from build123d import *

# Parameters (mm, degrees)
SKETCH1_W           = 110
SKETCH1_H           = 160
BOSS_EXTRUDE1_DEPTH = 3
SKETCH2_W           = 3
SKETCH2_H           = 15
BOSS_EXTRUDE2_DEPTH = 20
FILLET1_R           = 5
SKETCH3_R           = 3
CUT_EXTRUDE1_DEPTH  = 120
CUT_EXTRUDE2_DEPTH  = 10


with BuildPart() as part:
    # Sketch1 → Boss-Extrude1 (new body)
    with BuildSketch(Plane.XY):
        with Locations((55, 80)):
            Rectangle(SKETCH1_W, SKETCH1_H)
    extrude(amount=BOSS_EXTRUDE1_DEPTH)

    # Sketch2 → Boss-Extrude2 (add)
    with BuildSketch(Plane(origin=(0, 0, 0), x_dir=(-1, 0, 0), z_dir=(0, 0, -1))):
        with Locations((-4.5, 122.5)):
            Rectangle(SKETCH2_W, SKETCH2_H)
        with Locations((-4.5, 37.5)):
            Rectangle(SKETCH2_W, SKETCH2_H)
        with Locations((-105.5, 37.5)):
            Rectangle(SKETCH2_W, SKETCH2_H)
        with Locations((-105.5, 122.5)):
            Rectangle(SKETCH2_W, SKETCH2_H)
    extrude(amount=BOSS_EXTRUDE2_DEPTH)

    # Fillet1
    fillet1_edges = [part.edges().sort_by_distance(p)[0] for p in [
        (6, 122.5, 0),
        (6, 37.5, 0),
        (104, 37.5, 0),
        (104, 122.5, 0),
    ]]
    fillet(fillet1_edges, radius=FILLET1_R)

    # Sketch3 → Cut-Extrude1 (cut)
    with BuildSketch(Plane(origin=(107, 0, 0), x_dir=(0, 0, -1), z_dir=(1, 0, 0))):
        with Locations((10, 122.5)):
            Circle(SKETCH3_R)
        with Locations((10, 37.5)):
            Circle(SKETCH3_R)
    extrude(amount=-CUT_EXTRUDE1_DEPTH, mode=Mode.SUBTRACT)

    # Sketch4 → Cut-Extrude2 (cut)
    with BuildSketch(Plane(origin=(0, 0, 0), x_dir=(-1, 0, 0), z_dir=(0, 0, -1))):
        Polygon((-97.404603448, 115.083332467), (-71.456820791, 149.11710788), (-97.404603448, 149.11710788), align=None)
        Polygon((-39.377270954, 115.240473699), (-75.208928564, 132.650284128), (-97.404603448, 103.53786924), (-97.404603448, 79.025613644), align=None)
        Polygon((-12.834970583, 149.11710788), (-62.654412981, 149.11710788), (-70.879295193, 138.329141999), (-12.834970583, 110.126687653), align=None)
        Polygon((-12.834970583, 56.494500283), (-12.834970583, 102.344156626), (-31.943432736, 111.628536023), (-63.844562164, 91.719040132), align=None)
        Polygon((-70.31535921, 87.68061549), (-97.404603448, 70.774217299), (-97.404603448, 39.706571637), (-44.85383039, 70.098223458), align=None)
        Polygon((-78.83079022, 42.362019492), (-97.404603448, 31.620239081), (-97.404603448, 10.88289212), (-40.243023437, 10.88289212), align=None)
        Polygon((-12.834970583, 10.88289212), (-12.834970583, 47.98768369), (-38.481002615, 65.697483931), (-72.350817961, 46.109577315), (-29.169217126, 10.88289212), align=None)
    extrude(amount=-CUT_EXTRUDE2_DEPTH, mode=Mode.SUBTRACT)


solid = part.part
Work out the finished part from the listing and answer in its coordinate system (mm). A direction names the side the tool comes from. Give positions to 0.01 mm unless a question says otherwise; leave off trailing zeros. Write each loop counter-clockwise with the first axis right and the second up, starting at its lowest first coordinate (ties: lowest second). Pieces come first, ordered by that corner, then holes.
Q1. For a pull along X with two mould halves and no side action, classify faces 1 (the face through (102, 123, -1)), 2 (the face through (37, 149.117, 1)), 3 (the face through (4.521, 40.474, -9.609)), 4 (the face through (3, 34, -10)) as released by +X, released by -X, zero draft, split by the parting line, or undercut.
Answer:
face 1: undercut
face 2: undercut
face 3: zero draft
face 4: released by -X
Q2. The part is cut by section D-D on y = 141. Give the vertices of the cut face in (x, z).
Answer:
outline: (0, 0) - (12.83, 0) - (12.83, 3) - (0, 3) - close; (68.84, 0) - (77.65, 0) - (77.65, 3) - (68.84, 3) - close; (97.4, 0) - (110, 0) - (110, 3) - (97.4, 3) - close
Q3. The part is cut by section B-B on x = 22. Give the vertices of the cut face in (y, z).
Answer:
outline: (0, 0) - (10.88, 0) - (10.88, 3) - (0, 3) - close; (54.32, 0) - (62.82, 0) - (62.82, 3) - (54.32, 3) - close; (106.8, 0) - (114.58, 0) - (114.58, 3) - (106.8, 3) - close; (149.12, 0) - (160, 0) - (160, 3) - (149.12, 3) - close
Q4. A tool of negligible diameter and unlimited length cuts with its end or side. For faces 5 (the face through (87.988, 37.066, 1.479)), 6 (the face through (106, 45, -10)), 7 (the face through (4, 30, -10)), 8 (the face through (104, 37, -14)), from which of +Z, -Z, +X, -X, +Y, -Y can it reach the whole face along a straight path? Write none if from no direction.
Answer:
face 5: +Z, -Z
face 6: -Z, +X, -X
face 7: -Z, +X, -X, -Y
face 8: -Z, +Y, -Y
Q5. The part is cut by section A-A on z = -10. State how many separate pieces and enclosed holes the cut face has, and give its area (3 significant figures).
Answer:
separate pieces: 8
enclosed holes: 0
area: 108 mm2
Q6. Straight lines are drawn through the part: L1, parallel to Y at x = 104.9, z = -10; L2, parallel to X at y = 120, z = 1; L3, parallel to Z at x = 99, y = 55. For each, find the intervals that lie inside material, in ascending order.
Answer:
L1: y = 30 to 34.5, 40.5 to 45, 115 to 119.5, 125.5 to 130
L2: x = 0 to 12.83, 33.16 to 49.17, 84.85 to 93.66, 97.4 to 110
L3: z = 0 to 3
Q7. The part is cut by section C-C on z = -3. Give the vertices of the cut face in (x, y).
Answer:
outline: (3, 30) - (6.42, 30) - (6.42, 45) - (3, 45) - close; (3, 115) - (6.42, 115) - (6.42, 130) - (3, 130) - close; (103.58, 30) - (107, 30) - (107, 45) - (103.58, 45) - close; (103.58, 115) - (107, 115) - (107, 130) - (103.58, 130) - close
Q8. Given pin 1 (1.5 mm diameter, centred on x = 32, z = 1.5, fed in from -Y); pin 2 (1.5 mm diameter, centred on y = 127.5, z = -15.5, fed in from +X); pin 3 (2 mm diameter, centred on y = 116.5, z = -2, fed in from -X); pin 4 (4 mm diameter, centred on x = 103, z = -13, fed in from +Y), each flat-ended and moving along its own axis, determine where each tip first touches the part or whether it passes through.
Answer:
pin 1: stops at y = 0
pin 2: stops at x = 107
pin 3: stops at x = 3
pin 4: stops at y = 130
